Here's how the part is built. I have some questions about the finished solid (model axes, mm). Face numbers are marked on the shaded views. A direction names the side the tool comes from. Round coordinates to 2 decimals unless told otherwise and drop trailing zeros. Loops run counter-clockwise (first coordinate to the right, second up) from the corner with the lowest first, then second, coordinate; pieces in that order, holes last. Notation, with made-up numbers: (29, 7.25) -> (78, 7.25) arc R11 ccw to (78, 23.25) -> close; hole circle Ø1 at (-36.5, 10). An arc over 180 degrees is marked (long way). Use one line per item in the form item = value. Start each with the question number.
Item 1: If I drill on L1, parallel to Z at x = -8.5, y = -13.5; L2, parallel to Y at x = 6, z = 14; L3, parallel to Z at x = 5.5, y = -39, over which ranges is the centre line in solid material (lowest first)? Write a range as [from, to].
Item 2: If we section it at A-A (y = -23): Write out the boundary of the cut face in (x, z).
Item 3: If we section it at C-C (x = 0.25): Write out the boundary of the cut face in (y, z), then the cut area to 3 significant figures.
Item 4: Thinking about a two-plate mould opening in Z: for the marked faces 3, 4 and 5, which applies, released by +Z, released by -Z, zero draft, split by the parting line, or undercut?
Item 5: For the marked faces 1 and 2, which set-ups out of +Z, -Z, +X, -X, +Y, -Y let a thin tool reach every point of the face, with its end or its side?
Item 6: If we section it at B-B (z = -38.5): Write out the boundary of the cut face in (x, y), then the cut area to 3 significant figures.
Autodesk Fusion 360 part; units mm, degrees
sketch "Sketch1" plane through (0, 0, 0) normal (1, 0, 0) x (0, 1, 0)
  line L0 (-66.04, 63.5) -> (0, 63.5)
  line L1 (0, 63.5) -> (0, -63.5)
  line L2 (0, -63.5) -> (-66.04, -63.5)
  line L3 (-66.04, -63.5) -> (-66.04, 63.5)
  line L4 (-8.89, 54.61) -> (-40.64, 54.61)
  line L5 (-40.64, 54.61) -> (-40.64, -54.61)
  line L6 (-40.64, -54.61) -> (-8.89, -54.61)
  line L7 (-8.89, -54.61) -> (-8.89, 54.61)
  dimension "d1" = 127
  dimension "d2" = 31.75
  dimension "d3" = 8.89
  dimension "d4" = 8.89
  dimension "d5" = 25.4
  dimension "d6" = 8.89
extrude "Extrude1" add sketch "Sketch1" along normal mid plane 25.4
fillet "Fillet1" radius 12.7 1 edges at (0, -40.64, -54.61)
fillet "Fillet2" radius 12.7 1 edges at (0, -40.64, 54.61)
fillet "Fillet3" radius 19.05 1 edges at (0, -66.04, 63.5)
fillet "Fillet4" radius 19.05 1 edges at (0, -66.04, -63.5)
sketch "Sketch2" plane through (0, -66.04, 0) normal (0, -1, 0) x (1, 0, 0)
  line L0 (-12.7, -44.45) -> (12.7, -44.45)
  line L1 (12.7, -44.45) -> (12.7, 44.45)
  line L2 (12.7, 44.45) -> (-12.7, 44.45)
  line L3 (-12.7, 44.45) -> (-12.7, -44.45)
  line L4 (7.181, -50.5634) -> (7.181, 50.5634) construction
  line L5 (7.181, 50.5634) -> (-7.181, 50.5634) construction
  line L6 (-7.181, 50.5634) -> (-7.181, -50.5634) construction
  line L7 (-7.181, -50.5634) -> (7.181, -50.5634) construction
  dimension "d17" = 12.7
extrude "Extrude2" [suppressed]
fillet "Fillet5" radius 2.5 23 edges at (12.7, -8.89, 0) (0, -8.89, 54.61) (12.7, -18.415, -54.61) (12.7, -36.9203, -50.8903) (12.7, -40.64, 0) (12.7, -36.9203, 50.8903) (12.7, -18.415, 54.61) (-12.7, -8.89, 0) (-12.7, -18.415, 54.61) (-12.7, -36.9203, 50.8903) (-12.7, -40.64, 0) (-12.7, -36.9203, -50.8903) (-12.7, -18.415, -54.61) (12.7, -23.495, 63.5) (12.7, -60.4604, 57.9204) (12.7, -66.04, 0) (12.7, -60.4604, -57.9204) (12.7, -23.495, -63.5) (-12.7, -23.495, 63.5) (-12.7, -60.4604, 57.9204) (-12.7, -66.04, 0) (-12.7, -60.4604, -57.9204) (-12.7, -23.495, -63.5)
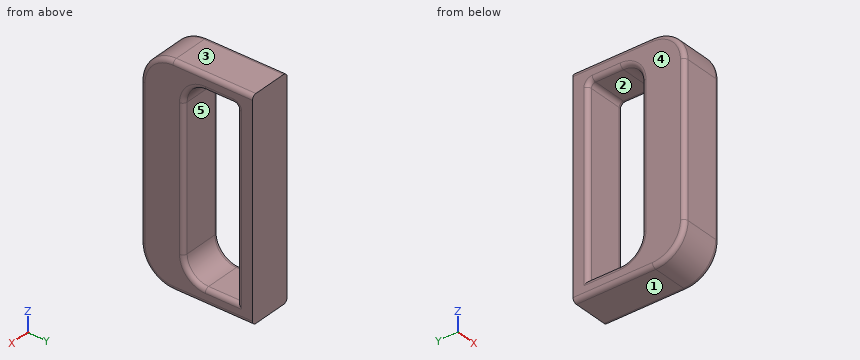
Values found:
q1.L1 = [-63.5, -54.61], [54.61, 63.5]
q1.L2 = [-66.04, -40.64], [-8.89, 0]
q1.L3 = [-63.5, -48.15], [48.15, 63.5]
q2.outline = (-12.7, -61) arc R2.5 ccw to (-10.2, -63.5) -> (10.2, -63.5) arc R2.5 ccw to (12.7, -61) -> (12.7, -57.11) arc R2.5 ccw to (10.2, -54.61) -> (-10.2, -54.61) arc R2.5 ccw to (-12.7, -57.11) -> close; (-12.7, 57.11) arc R2.5 ccw to (-10.2, 54.61) -> (10.2, 54.61) arc R2.5 ccw to (12.7, 57.11) -> (12.7, 61) arc R2.5 ccw to (10.2, 63.5) -> (-10.2, 63.5) arc R2.5 ccw to (-12.7, 61) -> close
q3.outline = (-66.04, -44.45) arc R19.05 ccw to (-46.99, -63.5) -> (0, -63.5) -> (0, 63.5) -> (-46.99, 63.5) arc R19.05 ccw to (-66.04, 44.45) -> close; hole (-40.64, -41.91) arc R12.7 ccw to (-27.94, -54.61) -> (-8.89, -54.61) -> (-8.89, 52.11) arc R2.5 ccw to (-11.39, 54.61) -> (-27.94, 54.61) arc R12.7 ccw to (-40.64, 41.91) -> close
q3.area = 4,830 mm2
q4.face_3 = released by +Z
q4.face_4 = zero draft
q4.face_5 = undercut
q5.face_1 = -Z, +X, -X, +Y, -Y
q5.face_2 = +X, -X
q6.outline = (-12.7, -63.54) arc R2.5 ccw to (-10.2, -66.04) -> (10.2, -66.04) arc R2.5 ccw to (12.7, -63.54) -> (12.7, -43.14) arc R2.5 ccw to (10.2, -40.64) -> (-10.2, -40.64) arc R2.5 ccw to (-12.7, -43.14) -> close; (-12.7, -6.39) arc R2.5 ccw to (-10.2, -8.89) -> (10.2, -8.89) arc R2.5 ccw to (12.7, -6.39) -> (12.7, 0) -> (-12.7, 0) -> close
q6.area = 863 mm2
